Part print with two shaded views. Sizes in mm from the minimum x, y, z corner. A direction names the side the tool comes from. Round coordinates to 2 decimals unless told otherwise and drop trailing zeros. Order: outer loops, then holes, each group sorted by start corner. A loop starts at its lowest first (then second) coordinate and runs counter-clockwise, first axis right, second up. Notation, with made-up numbers: (-29, -30.5) -> (-24, -30.5) arc R25 cw to (-24, -14.5) -> close; hole circle Ø11 at (59, 13.25). An arc over 180 degrees is marked (long way). Use a Markdown table: item, result. Add a question column.
Item 1: Probe L1, parallel to Y at x = 16, z = 14.5; L2, parallel to Y at x = 22.5, z = 36; L3, parallel to Z at x = 16, y = 27.2. List the from-to ranges inside material, lowest first.
Item 2: Two-plate mould, pull along X, no slides. Class the marked faces 1, 2 and 3: released by +X, released by -X, zero draft, split by the parting line, or undercut.
Item 3: Slice it at A-A, the plane x = 16. State how many separate pieces and enclosed holes the cut face has, plus the area to 3 significant figures.
Item 4: Slice it at B-B, the plane z = 10. Give the cut face in (x, y).
Item 5: 3-axis set-ups, long thin cutter, end or side, ignore diameter. For the marked faces 4 and 5: which of +Z, -Z, +X, -X, +Y, -Y reach the whole face in a straight line?
Item 6: Slice it at D-D, the plane z = 18. Give the cut face in (x, y), plus the area to 3 significant figures.
Item 7: Pin check, flat tips, straight feed: pin 1 (10 mm diameter, centred on y = 17.5, z = 21.5, fed in from -X); pin 2 (12.5 mm diameter, centred on x = 16, y = 16, fed in from -Z); pin 3 (1.3 mm diameter, centred on x = 7.5, y = 7.5, fed in from +Z). Stop position of each tip, or through.
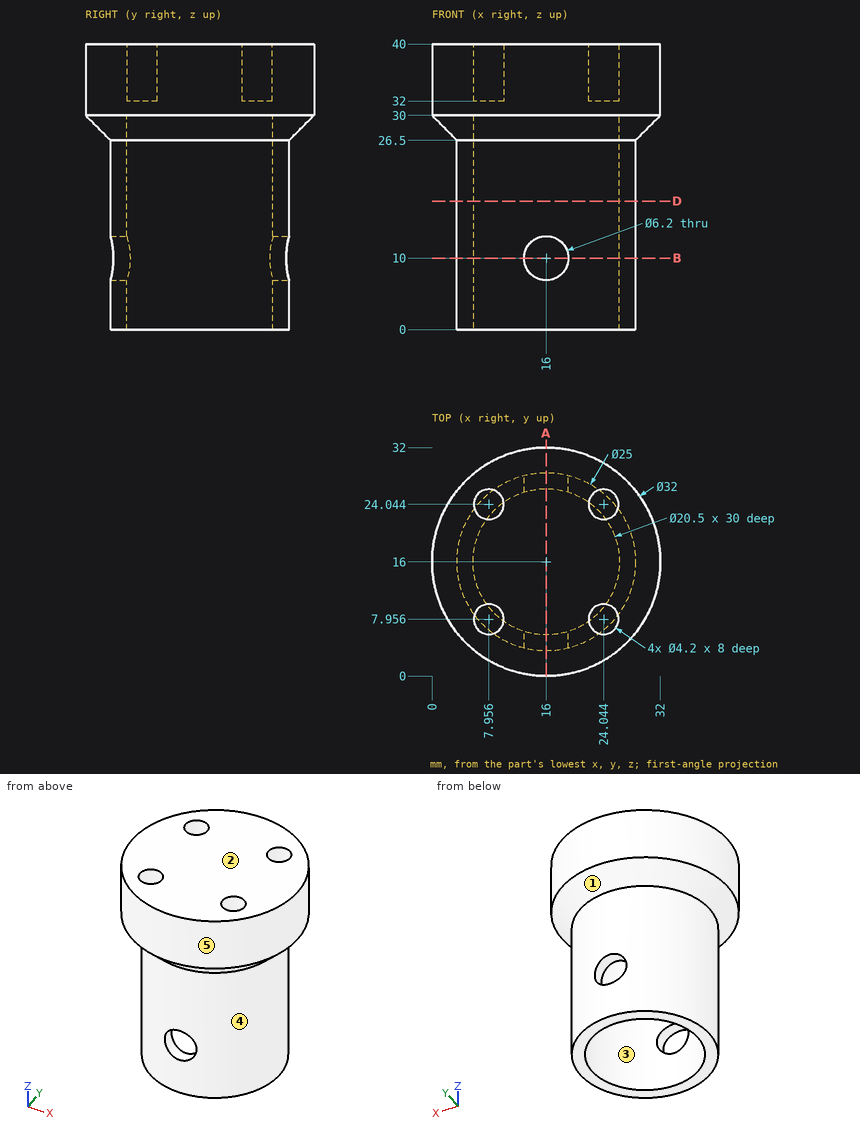
Check sheet entries:
| question | item | result |
|---|---|---|
| 1 | L1 | 3.5 to 5.75, 26.25 to 28.5 |
| 1 | L2 | 1.38 to 6.53, 9.38 to 22.62, 25.47 to 30.62 |
| 1 | L3 | 0 to 6.9, 13.1 to 40 |
| 2 | face 1 | split by the parting line |
| 2 | face 2 | zero draft |
| 2 | face 3 | undercut |
| 3 | separate pieces | 3 |
| 3 | enclosed holes | 0 |
| 3 | area | 439 mm2 |
| 4 | outline | (12.9, 3.89) -> (12.9, 6.23) arc R10.25 cw to (12.9, 25.77) -> (12.9, 28.11) arc R12.5 ccw to start; (19.1, 3.89) arc R12.5 ccw to (19.1, 28.11) -> (19.1, 25.77) arc R10.25 cw to (19.1, 6.23) -> close |
| 5 | face 4 | -Z |
| 5 | face 5 | +Z, -Z |
| 6 | outline | circle Ø25 at (16, 16); hole circle Ø20.5 at (16, 16) |
| 6 | area | 161 mm2 |
| 7 | pin 1 | x = 3.5 |
| 7 | pin 2 | z = 30 |
| 7 | pin 3 | z = 32 |
